Check sheet for the modelled part. Datum: model origin and axes. Units: mm. Round coordinates to 2 decimals unless told otherwise and drop trailing zeros. Order: outer loops, then holes, each group sorted by start corner. A loop starts at its lowest first (then second) coordinate and runs counter-clockwise, first axis right, second up.
Q1. Cross-section at A-A on y = 0. Record the cut outline in (x, z).
Q2. Scan lines: probe 1 along Y at (x, z) = (27.5, 0.85); probe 2 along X at (y, z) = (0.5, 0.2); probe 3 along X at (y, z) = (1, 0.1). Record each from-to range of solid material in increasing order.
Q3. Cross-section at B-B on x = 27.5. Record the cut outline in (y, z), then the cut area to 3 significant figures.
Q4. Mould release check, pull along Y, two halves, no side actions. Record for faces 1 (the cylindrical face through (29, 0, 1)), 2 (the cylindrical face through (-26, 0, 1)), 3 (the flat face through (0, 20, 1)), 4 (the flat face through (-30, 0, 1)): +Y half, -Y half, draft (parallel to the pull), parting line (faces both ways), or undercut.
from build123d import *

# Parameters (mm, degrees)
SKETCH1_W           = 60
SKETCH1_H           = 40
BOSS_EXTRUDE1_DEPTH = 2
CUT_EXTRUDE1_REACH  = 38.111
SKETCH2_R           = 1.5


with BuildPart() as part:
    # Sketch1 → Boss-Extrude1 (new body)
    with BuildSketch(Plane.XY):
        Rectangle(SKETCH1_W, SKETCH1_H)
    extrude(amount=BOSS_EXTRUDE1_DEPTH)

    # Sketch2 → Cut-Extrude1 (cut, up to next)
    with BuildSketch(Plane(origin=(0, 0, 0), x_dir=(-1, 0, 0), z_dir=(0, 0, -1)), mode=Mode.PRIVATE) as cut_extrude1_sk1:
        with Locations((27.5, 0)):
            Circle(SKETCH2_R)
    cut_extrude1_tool1 = extrude(cut_extrude1_sk1.sketch, amount=-CUT_EXTRUDE1_REACH, mode=Mode.PRIVATE) & part.part
    # Sketch2 → Cut-Extrude1 (cut, up to next)
    with BuildSketch(Plane(origin=(0, 0, 0), x_dir=(-1, 0, 0), z_dir=(0, 0, -1)), mode=Mode.PRIVATE) as cut_extrude1_sk2:
        with Locations((-27.5, 0)):
            Circle(SKETCH2_R)
    cut_extrude1_tool2 = extrude(cut_extrude1_sk2.sketch, amount=-CUT_EXTRUDE1_REACH, mode=Mode.PRIVATE) & part.part
    add(cut_extrude1_tool1.solids().sort_by_distance((-27.5, 0, 0))[0], mode=Mode.SUBTRACT)
    add(cut_extrude1_tool2.solids().sort_by_distance((27.5, 0, 0))[0], mode=Mode.SUBTRACT)


solid = part.part
Results found:
1. outline: (-30, 0) - (-29, 0) - (-29, 2) - (-30, 2) - close; (-26, 0) - (26, 0) - (26, 2) - (-26, 2) - close; (29, 0) - (30, 0) - (30, 2) - (29, 2) - close
2. probe 1: y = -20 to -1.5, 1.5 to 20
2. probe 2: x = -30 to -28.91, -26.09 to 26.09, 28.91 to 30
2. probe 3: x = -30 to -28.62, -26.38 to 26.38, 28.62 to 30
3. outline: (-20, 0) - (-1.5, 0) - (-1.5, 2) - (-20, 2) - close; (1.5, 0) - (20, 0) - (20, 2) - (1.5, 2) - close
3. area: 74.0 mm2
4. face 1: undercut
4. face 2: undercut
4. face 3: +Y half
4. face 4: draft
